```python
from build123d import *

# Parameters (mm, degrees)
F0_R     = 52.5
F0_R_2   = 1.75
F0_R_3   = 42.5
F1_DEPTH = 2
F0_R_4   = 20
F2_DEPTH = 7
F3_T     = -2
F4_R     = 10.25
F5_DEPTH = 25
F6_R     = 3.5
F7_DEPTH = 25


with BuildPart() as f1:
    # F0 (on Top) → F1 (new body)
    with BuildSketch(Plane.XY):
        Circle(F0_R)
        with Locations((0, -47.5)):
            Circle(F0_R_2, mode=Mode.SUBTRACT)
        with Locations((-47.5, 0)):
            Circle(F0_R_2, mode=Mode.SUBTRACT)
        Circle(F0_R_3, mode=Mode.SUBTRACT)
        with Locations((47.5, 0)):
            Circle(F0_R_2, mode=Mode.SUBTRACT)
        with Locations((0, 47.5)):
            Circle(F0_R_2, mode=Mode.SUBTRACT)
    extrude(amount=F1_DEPTH)

    # F0 (on Top) → F2 (join)
    with BuildSketch(Plane.XY):
        Circle(F0_R_3)
        Circle(F0_R_4, mode=Mode.SUBTRACT)
    extrude(amount=F2_DEPTH)

    # F3
    f3_openings = [f1.faces().sort_by_distance(p)[0] for p in [
        (-41.297918, 0, 7),
    ]]
    offset(amount=F3_T, openings=f3_openings, kind=Kind.INTERSECTION)

    # F4 (on face) → F5 (cut)
    with BuildSketch(Plane.XY.offset(2)):
        with Locations((0, 31.25)):
            Circle(F4_R)
        with Locations((-31.25, 0)):
            Circle(F4_R)
        with Locations((0, -31.25)):
            Circle(F4_R)
        with Locations((31.25, 0)):
            Circle(F4_R)
    extrude(amount=F5_DEPTH, mode=Mode.SUBTRACT)

    # F6 (on face) → F7 (cut)
    with BuildSketch(Plane.XY.offset(2)):
        with Locations((-18.4997347846, -18.269094474)):
            Circle(F6_R)
    extrude(amount=-F7_DEPTH, mode=Mode.SUBTRACT)


solid = f1.part
```
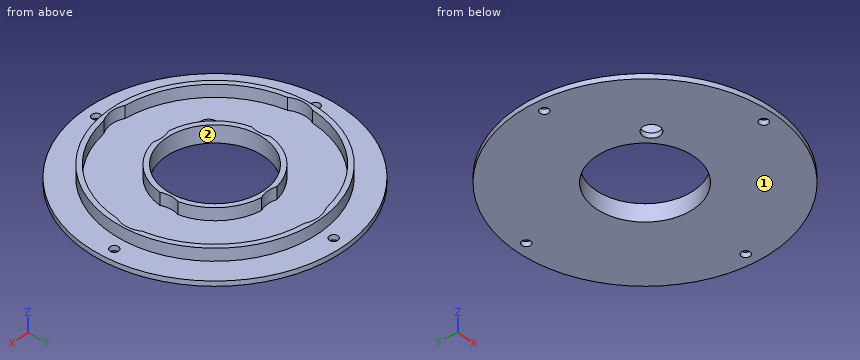
Can you work these out from the model? Positions are in its coordinate system, mm. Face numbers are marked on the shaded views. Coordinates: 2 decimals unless noted, no trailing zeros. Loops run counter-clockwise (first coordinate to the right, second up) from the corner with the lowest first, then second, coordinate; pieces in that order, holes last. Notation, with made-up numbers: (72.5, 76) -> (83.5, 76) arc R16 cw to (83.5, 99) -> close; hole circle Ø3 at (-11, -31). An arc over 180 degrees is marked (long way). Put each result on its own line as item: value. Start each with the question number.
Q1. If I drill on line 1 (Y direction, x = 0, z = 0.45); line 2 (Y direction, x = 0, z = 3); line 3 (X direction, y = 1, z = 5.75), over which ranges is the centre line in solid material (lowest first)? Write a range as [from, to].
Q2. I want a section at B-B (y = 0). Write out the boundary of the cut face in (x, z), plus the area to 3 significant figures.
Q3. I'm going to push flat-ended pins straight in: P1, Ø5.5, axis at x = 47.5, y = 0, coming from the +Z side; P2, Ø3, axis at x = 0, y = -47.5, coming from the +Z side; P3, Ø2, axis at y = 8.5, z = 4, coming from the +X side; P4, Ø2, axis at x = 33.5, z = 0.5, coming from the -Y side. Where does each tip first touch, or does it pass through?
Q4. I want a section at A-A (z = 5.25). Write out the boundary of the cut face in (x, y), plus the area to 3 significant figures.
Q5. Thinking about a two-plate mould opening in X: for the marked faces 1 and 2, which applies, pulls with the +X half, pulls with the -X half, needs draft (parallel to the pull), parting line crosses it, or undercut?
Q6. I want a section at D-D (x = 17). Write out the boundary of the cut face in (y, z), plus the area to 3 significant figures.
Taken from the geometry:
1. line 1: y = [-52.5, -49.25], [-45.75, -20], [20, 45.75], [49.25, 52.5]
1. line 2: y = [-42.5, -41.5], [-21, -20], [20, 21], [41.5, 42.5]
1. line 3: x = [-42.49, -41.45], [-21.05, -19.97], [19.97, 21.05], [41.45, 42.49]
2. outline: (-52.5, 0) -> (-49.25, 0) -> (-49.25, 2) -> (-52.5, 2) -> close; (-45.75, 0) -> (-20, 0) -> (-20, 7) -> (-21, 7) -> (-21, 2) -> (-41.5, 2) -> (-41.5, 7) -> (-42.5, 7) -> (-42.5, 2) -> (-45.75, 2) -> close; (20, 0) -> (45.75, 0) -> (45.75, 2) -> (42.5, 2) -> (42.5, 7) -> (41.5, 7) -> (41.5, 2) -> (21, 2) -> (21, 7) -> (20, 7) -> close; (49.25, 0) -> (52.5, 0) -> (52.5, 2) -> (49.25, 2) -> close
2. area: 136 mm2
3. P1: stops at z = 2
3. P2: passes through
3. P3: stops at x = 41.83
3. P4: stops at y = -41.23
4. outline: circle Ø85 at (0, 0); (-21.69, -3.69) arc R22 ccw to (-3.69, -21.69) arc R10.25 cw to (3.69, -21.69) arc R22 ccw to (21.69, -3.69) arc R10.25 cw to (21.69, 3.69) arc R22 ccw to (3.69, 21.69) arc R10.25 cw to (-3.69, 21.69) arc R22 ccw to (-21.69, 3.69) arc R10.25 cw to start; hole (-40.19, -5.02) arc R40.5 ccw to (-5.02, -40.19) arc R10.25 ccw to (5.02, -40.19) arc R40.5 ccw to (40.19, -5.02) arc R10.25 ccw to (40.19, 5.02) arc R40.5 ccw to (5.02, 40.19) arc R10.25 ccw to (-5.02, 40.19) arc R40.5 ccw to (-40.19, 5.02) arc R10.25 ccw to start; hole circle Ø40 at (0, 0)
4. area: 738 mm2
5. face 1: needs draft
5. face 2: undercut
6. outline: (-49.67, 0) -> (-10.54, 0) -> (-10.54, 7) -> (-13.96, 7) -> (-13.96, 2) -> (-36.76, 2) -> (-36.76, 7) -> (-38.95, 7) -> (-38.95, 2) -> (-49.67, 2) -> close; (10.54, 0) -> (49.67, 0) -> (49.67, 2) -> (38.95, 2) -> (38.95, 7) -> (36.76, 7) -> (36.76, 2) -> (13.96, 2) -> (13.96, 7) -> (10.54, 7) -> close
6. area: 213 mm2
